Geometry: see drawing. Coordinates: mm, zero at the bounding-box minimum. Coordinates: 2 decimals unless noted, no trailing zeros. Order: outer loops, then holes, each group sorted by start corner. A loop starts at its lowest first (then second) coordinate and runs counter-clockwise, first axis right, second up.
Item 1: Section A-A on x = 25.4. Return the cut outline in (y, z) (1 decimal).
Item 2: Ray query, line 1 (Y direction, x = 25.4, z = 1.55); line 2 (Y direction, x = 26, z = 1.45). Return the intervals inside material, ascending.
Item 3: Section B-B on y = 203.2. Return the cut outline in (x, z) (1 decimal), then the cut area to 3 significant figures.
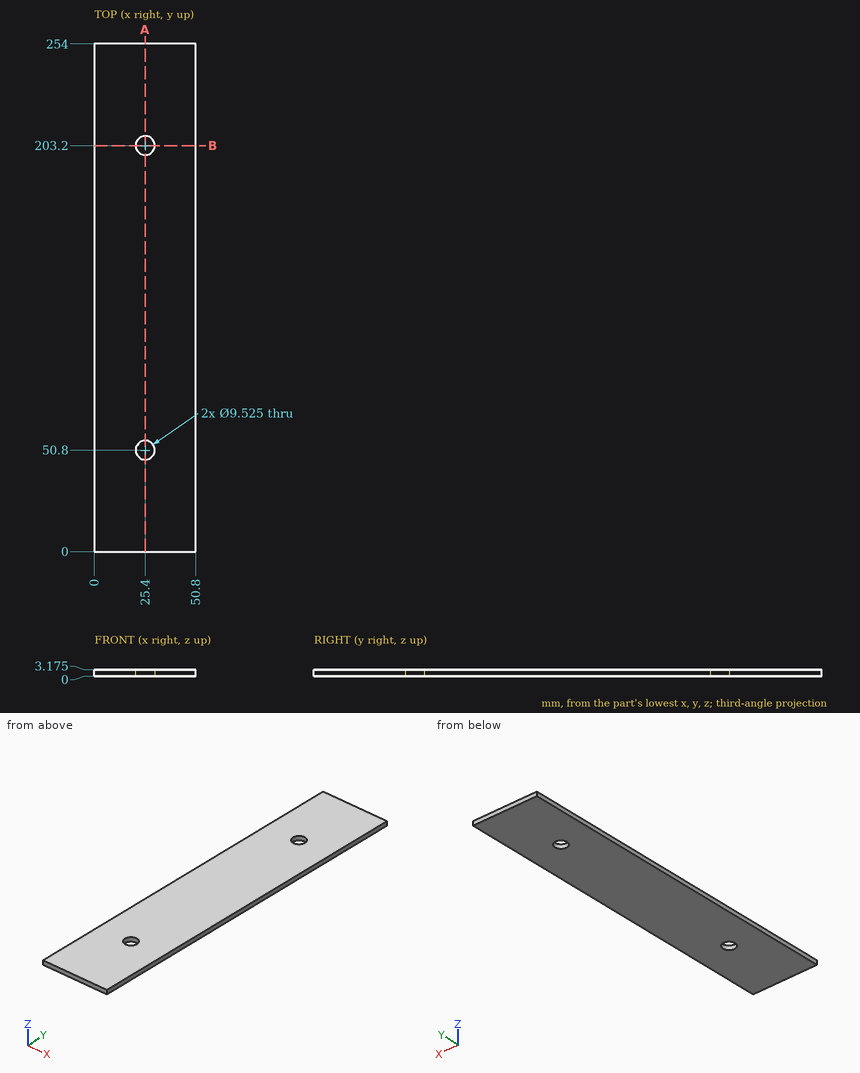
Answer list:
1. outline: (0, 0) - (46, 0) - (46, 3.2) - (0, 3.2) - close; (55.6, 0) - (198.4, 0) - (198.4, 3.2) - (55.6, 3.2) - close; (208, 0) - (254, 0) - (254, 3.2) - (208, 3.2) - close
2. line 1: y = 0 to 46.04, 55.56 to 198.44, 207.96 to 254
2. line 2: y = 0 to 46.08, 55.52 to 198.48, 207.92 to 254
3. outline: (0, 0) - (20.6, 0) - (20.6, 3.2) - (0, 3.2) - close; (30.2, 0) - (50.8, 0) - (50.8, 3.2) - (30.2, 3.2) - close
3. area: 131 mm2
